Autodesk Inventor part; units mm, degrees
ref_plane "YZ Plane" through (0, 0, 0) normal (1, 0, 0) x (0, 1, 0)
ref_plane "XZ Plane" through (0, 0, 0) normal (0, 1, 0) x (-1, 0, 0)
ref_plane "XY Plane" through (0, 0, 0) normal (0, 0, 1) x (1, 0, 0)
sketch "Sketch1" plane through (0, 0, 0) normal (0, 1, 0) x (-1, 0, 0)
  line L0 (-26.67, -28.76) -> (26.67, -28.76)
  line L1 (26.67, -28.76) -> (26.67, 28.76)
  line L2 (26.67, 28.76) -> (-26.67, 28.76)
  line L3 (-26.67, 28.76) -> (-26.67, -28.76)
  line L4 (-26.67, -28.76) -> (26.67, 28.76) construction
  line L5 (26.67, -28.76) -> (-26.67, 28.76) construction
  circle A0 centre (-24.13, 25.85) radius 1.5
  circle A1 centre (24.13, 24.58) radius 1.5
  circle A2 centre (-19.05, -26.25) radius 1.5
  point P0 (0, 0)
  point P1 (0, 0)
  dimension "d0" = 53.34
  dimension "d1" = 57.52
  dimension "d2" = 3
  dimension "d3" = 3
  dimension "d4" = 3
  dimension "d5" = 2.54
  dimension "d6" = 2.91
  dimension "d7" = 50.8
  dimension "d8" = 4.18
  dimension "d9" = 2.51
  dimension "d10" = 7.62
extrude "Extrusion1" add sketch "Sketch1" along normal blind 1.5
sketch "Sketch2" plane through (0, 1.5, 0) normal (0, 1, 0) x (1, 0, 0)
  line L0 (-26.67, 28.76) -> (-26.67, -28.76)
  line L1 (-26.67, -28.76) -> (26.67, -28.76)
  line L2 (26.67, -28.76) -> (26.67, 28.76)
  line L3 (26.67, 28.76) -> (-26.67, 28.76)
  circle A0 centre (24.13, -25.85) radius 1.5
  circle A1 centre (-24.13, -24.58) radius 1.5
  circle A2 centre (19.05, 26.25) radius 1.5
  line L4 (-26.67, -28.76) -> (26.67, -28.76)
  line L5 (0, -28.76) -> (0, 28.76)
  line L6 (9.3688, 25.76) -> (-9.3688, 25.76)
  line L7 (-9.3688, 25.76) -> (-9.3688, 7.4756)
  line L8 (-9.3688, 7.4756) -> (9.3688, 7.4756)
  line L9 (9.3688, 7.4756) -> (9.3688, 25.76)
  line L10 (9.3688, 25.76) -> (-9.3688, 7.4756) construction
  line L11 (-9.3688, 25.76) -> (9.3688, 7.4756) construction
  point P0 (0, 0)
  point P1 (0, 16.6178)
  dimension "d13" = 36.0388
  dimension "d14" = 3
extrude "Extrusion2" add sketch "Sketch2" along normal blind 3 contours L6 L9 L8 L5 | L5 L8 L7 L6
sketch "Sketch3" plane through (0, 1.5, 0) normal (0, 1, 0) x (1, 0, 0)
  line L0 (9.3688, 25.76) -> (9.3688, 7.4756)
  line L1 (9.3688, 7.4756) -> (-9.3688, 7.4756)
  line L2 (-9.3688, 7.4756) -> (-9.3688, 25.76)
  line L3 (-9.3688, 25.76) -> (9.3688, 25.76)
  line L4 (-26.67, 28.76) -> (-26.67, -28.76)
  line L5 (-26.67, -28.76) -> (26.67, -28.76)
  line L6 (26.67, -28.76) -> (26.67, 28.76)
  line L7 (26.67, 28.76) -> (-26.67, 28.76)
  circle A0 centre (24.13, -25.85) radius 1.5
  circle A1 centre (-24.13, -24.58) radius 1.5
  circle A2 centre (19.05, 26.25) radius 1.5
  circle A3 centre (24.13, -25.85) radius 1.5
  line L8 (24.13, -25.85) -> (24.13, 28.76)
  line L9 (26.67, 28.76) -> (-26.67, 28.76)
  line L10 (-24.13, -24.58) -> (-24.13, 28.76)
  line L11 (24.88, 24.099) -> (23.38, 24.099)
  line L12 (23.38, 24.099) -> (23.38, -14.4594)
  line L13 (23.38, -14.4594) -> (24.88, -14.4594)
  line L14 (24.88, -14.4594) -> (24.88, 24.099)
  line L15 (24.88, 24.099) -> (23.38, -14.4594) construction
  line L16 (23.38, 24.099) -> (24.88, -14.4594) construction
  line L17 (-24.88, 21.2829) -> (-23.38, 21.2829)
  line L18 (-23.38, 21.2829) -> (-23.38, -21.2829)
  line L19 (-23.38, -21.2829) -> (-24.88, -21.2829)
  line L20 (-24.88, -21.2829) -> (-24.88, 21.2829)
  line L21 (-24.88, 21.2829) -> (-23.38, -21.2829) construction
  line L22 (-23.38, 21.2829) -> (-24.88, -21.2829) construction
  point P0 (0, 0)
  point P1 (24.13, 4.8198)
  point P2 (-24.13, 0)
  dimension "d17" = 1.5
  dimension "d18" = 1.5
extrude "Extrusion3" add sketch "Sketch3" along normal blind 6 contours L11 L14 L13 L8 | L8 L13 L12 L11 | L17 L18 L19 L10 | L10 L19 L20 L17
sketch "Sketch4" plane through (0, 4.5, 0) normal (0, 1, 0) x (1, 0, 0)
  line L0 (9.3688, 25.76) -> (-9.3688, 25.76)
  line L1 (-9.3688, 25.76) -> (-9.3688, 7.4756)
  line L2 (-9.3688, 7.4756) -> (9.3688, 7.4756)
  line L3 (9.3688, 7.4756) -> (9.3688, 25.76)
  line L4 (4.8688, 11.9756) -> (-4.8688, 11.9756)
  line L5 (-4.8688, 11.9756) -> (-4.8688, 21.26)
  line L6 (-4.8688, 21.26) -> (4.8688, 21.26)
  line L7 (4.8688, 21.26) -> (4.8688, 11.9756)
  point P0 (0, 0)
  dimension "d21" = 4.5
extrude "Extrusion4" cut sketch "Sketch4" against normal blind 2 contours L4 L5 L6 L7
chamfer "Chamfer1" distance 2 angle 45 4 edges at (0, 4.5, -11.9756) (-4.8688, 4.5, -16.6178) (0, 4.5, -21.26) (4.8688, 4.5, -16.6178)
sketch "Sketch5" plane through (0, 1.5, 0) normal (0, 1, 0) x (1, 0, 0)
  line L0 (-26.67, -28.76) -> (26.67, -28.76)
  line L1 (-16.2954, -28.76) -> (-12.7903, -22.5498)
  line L2 (-12.7903, -22.5498) -> (0, -22.5498)
  line L3 (12.7903, -22.5498) -> (16.2954, -28.76)
  line L4 (0, -28.76) -> (0, -13.7349)
  line L5 (0, -22.5498) -> (12.7903, -22.5498)
  point P0 (0, 0)
extrude "Extrusion5" cut sketch "Sketch5" against normal through all
fillet "Fillet1" radius 2 8 edges at (26.67, 0.75, -28.76) (-26.67, 0.75, -28.76) (-26.67, 0.75, 28.76) (-16.2954, 0.75, 28.76) (-12.7903, 0.75, 22.5498) (12.7903, 0.75, 22.5498) (16.2954, 0.75, 28.76) (26.67, 0.75, 28.76)
fillet "Fillet2" radius 2 4 edges at (9.3688, 3, -25.76) (9.3688, 3, -7.4756) (-9.3688, 3, -7.4756) (-9.3688, 3, -25.76)
properties part number "mti_3"
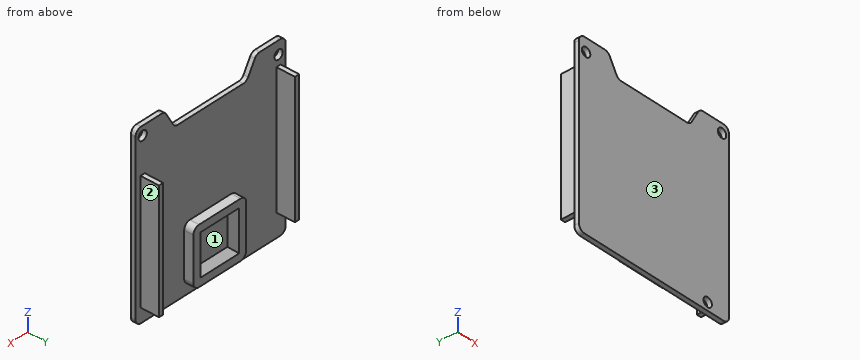
Build history of the part. All positions in model axes, mm. Face numbers are marked on the shaded views. Coordinates: 2 decimals unless noted, no trailing zeros. Write each loop counter-clockwise with the first axis right and the second up, starting at its lowest first coordinate (ties: lowest second). Pieces come first, ordered by that corner, then holes.
(1) Cut at A-A on x = 19.05. List the corners of the cut face in (y, z), and give its area (3 significant figures).
(2) Cut at C-C on x = -8.5. List the corners of the cut face in (y, z), and give its area (3 significant figures).
(3) Cut at D-D on z = 4.5. List the corners of the cut face in (x, y), and give its area (3 significant figures).
(4) Mould opens along X. For the marked faces 1, 2 and 3 say: pulls with the +X half, pulls with the -X half, needs draft (parallel to the pull), parting line crosses it, or undercut.
(5) Drill centre lines: line 1 (Z direction, x = 24.13, y = 1); line 2 (Z direction, x = 19.05, y = 1.15); line 3 (X direction, y = 3, z = -2). Where is each one in solid material? Low to high.
(6) Pin check, flat tips, straight feed: pin 1 Ø10 at (x, z) = (-12.5, 5.5) entering from -Y; pin 2 Ø10 at (x, z) = (4, -22) entering from +Y; pin 3 Ø3 at (y, z) = (6.5, 7.5) entering from +X; pin 4 Ø1 at (x, y) = (-9, 3) entering from +Z. Stop position of each tip, or through.
Working result:
1. outline: (0, -28.76) - (1.5, -28.76) - (1.5, -27.75) - (0, -27.75) - close; (0, -24.75) - (1.5, -24.75) - (1.5, 28.76) - (0, 28.76) - close
1. area: 81.8 mm2
2. outline: (0, -28.76) - (1.5, -28.76) - (1.5, -25.41) - (4.5, -25.41) - (4.5, -7.83) - (1.5, -7.83) - (1.5, 22.55) - (0, 22.55) - close
2. area: 130 mm2
3. outline: (-26.67, 0) - (26.67, 0) - (26.67, 1.5) - (24.88, 1.5) - (24.88, 7.5) - (23.38, 7.5) - (23.38, 1.5) - (-23.38, 1.5) - (-23.38, 7.5) - (-24.88, 7.5) - (-24.88, 1.5) - (-26.67, 1.5) - close
3. area: 98.0 mm2
4. face 1: undercut
4. face 2: pulls with the +X half
4. face 3: needs draft
5. line 1: z = -28.76 to 24.35, 27.35 to 28.76
5. line 2: z = -28.76 to -27.75, -24.75 to 28.76
5. line 3: x = -24.88 to -23.38, 23.38 to 24.88
6. pin 1: stops at y = 0
6. pin 2: stops at y = 4.5
6. pin 3: stops at x = 24.88
6. pin 4: stops at z = -7.83
